The drawing under review shows one solid part. Ordinate dimensions are in mm from its lowest x, y, z. Round coordinates to 2 decimals unless told otherwise and drop trailing zeros. Order: outer loops, then holes, each group sorted by start corner. A loop starts at its lowest first (then second) coordinate and runs counter-clockwise, first axis right, second up. Notation, with made-up numbers: M 31,65 L 61,65 A17 cw 61,96 Z; hole C 53,1.5 d7. An arc over 180 degrees is marked long. Answer as a JSON object with one key per item and string values. Group by question number.
1. Add section A-A on x = 39.5. State the section outline as (y, z) points, and give its area (3 significant figures).
2. To check wall thickness, follow probe 1 along X at (y, z) = (13.5, 2.25); probe 2 along Y at (x, z) = (22, 0.9). State the ranges of each line that lie inside material, in increasing order. Write a range as [from, to].
3. Add section B-B on z = 1.65. State the section outline as (x, y) points, and give its area (3 significant figures).
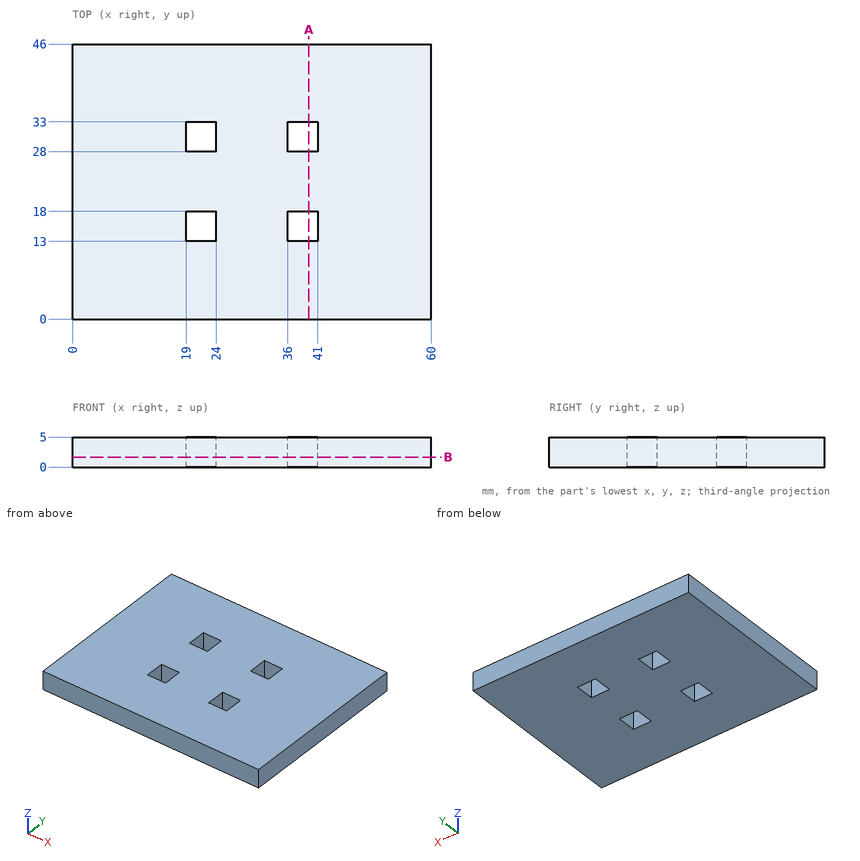
Recorded:
{
 "1": {"outline": "M 0,0 L 13,0 L 13,5 L 0,5 Z; M 18,0 L 28,0 L 28,5 L 18,5 Z; M 33,0 L 46,0 L 46,5 L 33,5 Z", "area": "180 mm²"},
 "2": {"probe 1": "x = [0, 19], [24, 36], [41, 60]", "probe 2": "y = [0, 13], [18, 28], [33, 46]"},
 "3": {"outline": "M 0,0 L 60,0 L 60,46 L 0,46 Z; hole M 19,13 L 24,13 L 24,18 L 19,18 Z; hole M 19,28 L 24,28 L 24,33 L 19,33 Z; hole M 36,13 L 41,13 L 41,18 L 36,18 Z; hole M 36,28 L 41,28 L 41,33 L 36,33 Z", "area": "2,660 mm²"}
}
